Check sheet for the drawn part. Datum: minimum x, y, z corner. Units: mm. A direction names the side the tool comes from. Coordinates: 2 decimals unless noted, no trailing zeros. Loops run counter-clockwise (first coordinate to the right, second up) from the corner with the lowest first, then second, coordinate; pieces in that order, holes last. Notation, with made-up numbers: (18.5, 31) - (45.5, 31) arc R21 cw to (45.5, 70) - close; hole circle Ø2 at (-23.75, -34.5). An arc over 180 degrees is marked (long way). Write item = value, one per line. Start each with the question number.
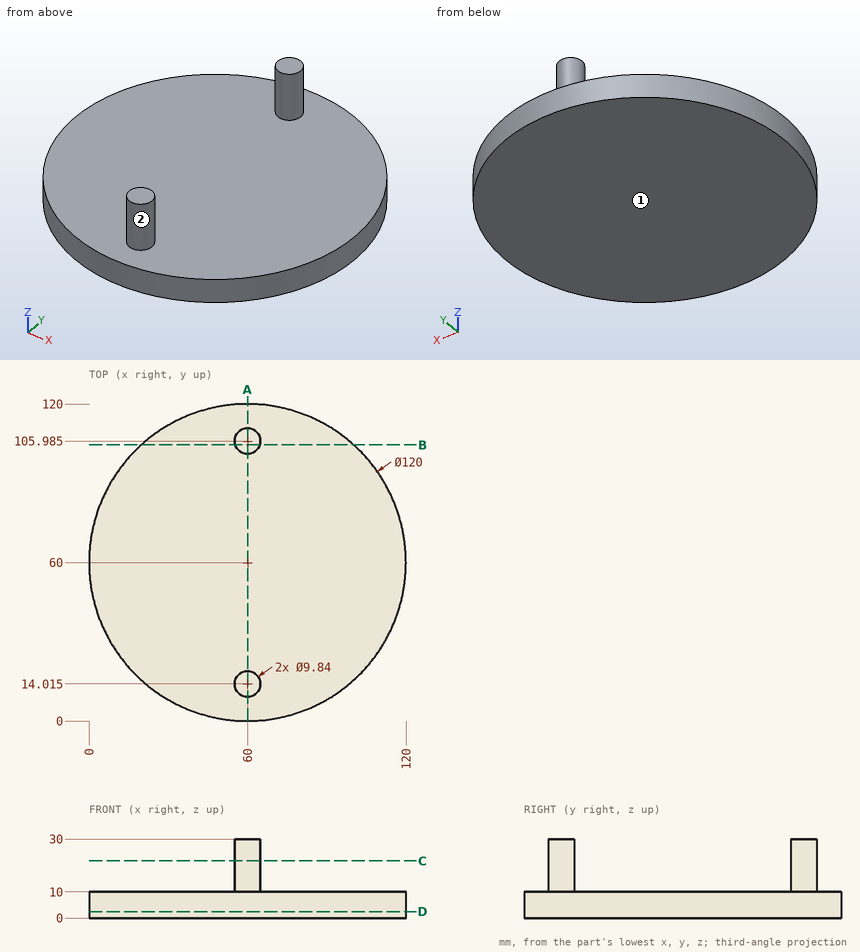
(1) Scan lines: line 1 (Z direction, x = 24, y = 103); line 2 (X direction, y = 112.5, z = 5.5); line 3 (X direction, y = 14.5, z = 5). Record each from-to range of solid material in increasing order.
(2) Tool access check on the marked faces 1 and 2. Record the directions out of +Z, -Z, +X, -X, +Y, -Y that give a thin tool (end or side, any length) a straight path to the whole face; none if there is none.
(3) Sectioned sample at A-A on x = 60. Enter the section's corners in (y, z) (3 decimals).
(4) Sectioned sample at B-B on y = 104.5. Enter the section's corners in (x, z).
(5) Depth check by flat-ended pin: pin 1 (10 mm diameter, centred on x = 47.5, z = 12, fed in from -Y); pin 2 (2 mm diameter, centred on x = 97.5, y = 40.5, fed in from +Z); pin 3 (5 mm diameter, centred on x = 64, z = 13.5, fed in from -Y). Enter the tip coordinate at first touch or a pass-through.
(6) Sectioned sample at C-C on z = 21.75. Enter the section's corners in (x, y) (3 decimals).
(7) Sectioned sample at D-D on z = 2.5. Enter the section's corners in (x, y).
Working result:
q1.line_1 = 0 to 10
q1.line_2 = 30.95 to 89.05
q1.line_3 = 20.89 to 99.11
q2.face_1 = -Z, +X, -X, +Y, -Y
q2.face_2 = +Z
q3.outline = (0, 0) - (120, 0) - (120, 10) - (110.905, 10) - (110.905, 30) - (101.065, 30) - (101.065, 10) - (18.935, 10) - (18.935, 30) - (9.095, 30) - (9.095, 10) - (0, 10) - close
q4.outline = (19.75, 0) - (100.25, 0) - (100.25, 10) - (64.69, 10) - (64.69, 30) - (55.31, 30) - (55.31, 10) - (19.75, 10) - close
q5.pin_1 = 0.52
q5.pin_2 = 10
q5.pin_3 = 9.33
q6.outline = circle Ø9.84 at (60, 14.015); circle Ø9.84 at (60, 105.985)
q7.outline = circle Ø120 at (60, 60)
